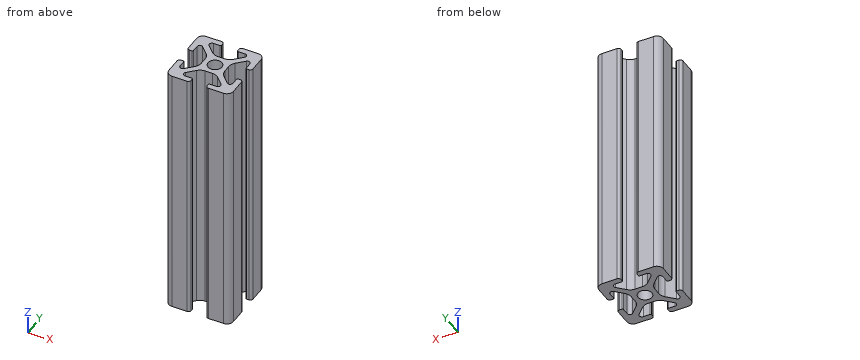
Autodesk Inventor part; units mm, degrees
ref_plane "Startebene" through (0, 0, 0) normal (0, 0, 1) x (1, 0, 0)
ref_plane "Endebene" through (0, 0, 80) normal (0, 0, 1) x (1, 0, 0)
ref_plane "YZ Plane" through (0, 0, 0) normal (1, 0, 0) x (0, 1, 0)
ref_plane "Startebene" through (0, 0, 0) normal (0, 0, 1) x (1, 0, 0)
ref_plane "Endebene" through (0, 0, 80) normal (0, 0, 1) x (1, 0, 0)
sketch "Skizze" plane through (0, 0, 0) normal (0, 0, 1) x (1, 0, 0)
  arc A0 (-4.5287, -3.2559) -> (-3.65, -1.1346) centre (-6.65, -1.1346) ccw
  line L0 (-3.65, -1.1346) -> (-3.65, 1.1346)
  circle A1 centre (0, 0) radius 2.15
  line L1 (1.1346, -3.65) -> (-1.1346, -3.65)
  arc A2 (-1.1346, -3.65) -> (-3.2559, -4.5287) centre (-1.1346, -6.65) ccw
  line L2 (-6.779, -5.5062) -> (-4.5287, -3.2559)
  line L3 (-3.2559, -4.5287) -> (-5.5062, -6.779)
  arc A3 (-2.5, -8.5) -> (-2.8, -8.2) centre (-2.8, -8.5) ccw
  line L4 (-2.5, -8.5) -> (-2.5, -9.2)
  line L5 (-4.9176, -8.2) -> (-2.8, -8.2)
  arc A4 (-5.5062, -6.779) -> (-4.9176, -8.2) centre (-4.9176, -7.3676) ccw
  arc A5 (-3.3, -10) -> (-2.5, -9.2) centre (-3.3, -9.2) ccw
  line L6 (-3.3, -10) -> (-8, -10)
  line L7 (10, -3.3) -> (10, -8)
  line L8 (5.5062, -6.779) -> (3.2559, -4.5287)
  arc A6 (6.779, -5.5062) -> (8.2, -4.9176) centre (7.3676, -4.9176) ccw
  arc A7 (3.2559, -4.5287) -> (1.1346, -3.65) centre (1.1346, -6.65) ccw
  line L9 (4.5287, -3.2559) -> (6.779, -5.5062)
  arc A8 (3.65, -1.1346) -> (4.5287, -3.2559) centre (6.65, -1.1346) ccw
  arc A9 (8.5, -2.5) -> (8.2, -2.8) centre (8.5, -2.8) ccw
  line L10 (3.65, 1.1346) -> (3.65, -1.1346)
  line L11 (8.5, -2.5) -> (9.2, -2.5)
  arc A10 (10, -3.3) -> (9.2, -2.5) centre (9.2, -3.3) ccw
  line L12 (8.2, -4.9176) -> (8.2, -2.8)
  line L13 (2.5, 8.5) -> (2.5, 9.2)
  arc A11 (2.5, 8.5) -> (2.8, 8.2) centre (2.8, 8.5) ccw
  arc A12 (1.1346, 3.65) -> (3.2559, 4.5287) centre (1.1346, 6.65) ccw
  line L14 (-1.1346, 3.65) -> (1.1346, 3.65)
  arc A13 (3.3, 10) -> (2.5, 9.2) centre (3.3, 9.2) ccw
  line L15 (4.9176, 8.2) -> (2.8, 8.2)
  arc A14 (4.5287, 3.2559) -> (3.65, 1.1346) centre (6.65, 1.1346) ccw
  line L16 (3.2559, 4.5287) -> (5.5062, 6.779)
  arc A15 (5.5062, 6.779) -> (4.9176, 8.2) centre (4.9176, 7.3676) ccw
  line L17 (6.779, 5.5062) -> (4.5287, 3.2559)
  line L18 (3.3, 10) -> (8, 10)
  arc A16 (10, 8) -> (8, 10) centre (8, 8) ccw
  line L19 (8.2, 2.8) -> (8.2, 4.9176)
  line L20 (10, 8) -> (10, 3.3)
  arc A17 (8.2, 4.9176) -> (6.779, 5.5062) centre (7.3676, 4.9176) ccw
  line L21 (-2.8, 8.2) -> (-4.9176, 8.2)
  line L22 (-2.5, 9.2) -> (-2.5, 8.5)
  arc A18 (-2.5, 9.2) -> (-3.3, 10) centre (-3.3, 9.2) ccw
  arc A19 (-2.8, 8.2) -> (-2.5, 8.5) centre (-2.8, 8.5) ccw
  arc A20 (-3.65, 1.1346) -> (-4.5287, 3.2559) centre (-6.65, 1.1346) ccw
  arc A21 (-3.2559, 4.5287) -> (-1.1346, 3.65) centre (-1.1346, 6.65) ccw
  arc A22 (4.9176, -8.2) -> (5.5062, -6.779) centre (4.9176, -7.3676) ccw
  arc A23 (8, -10) -> (10, -8) centre (8, -8) ccw
  line L23 (2.8, -8.2) -> (4.9176, -8.2)
  line L24 (8, -10) -> (3.3, -10)
  arc A24 (2.8, -8.2) -> (2.5, -8.5) centre (2.8, -8.5) ccw
  arc A25 (2.5, -9.2) -> (3.3, -10) centre (3.3, -9.2) ccw
  line L25 (2.5, -9.2) -> (2.5, -8.5)
  arc A26 (8.2, 2.8) -> (8.5, 2.5) centre (8.5, 2.8) ccw
  line L26 (9.2, 2.5) -> (8.5, 2.5)
  arc A27 (9.2, 2.5) -> (10, 3.3) centre (9.2, 3.3) ccw
  arc A28 (-4.9176, 8.2) -> (-5.5062, 6.779) centre (-4.9176, 7.3676) ccw
  line L27 (-8, 10) -> (-3.3, 10)
  line L28 (-5.5062, 6.779) -> (-3.2559, 4.5287)
  arc A29 (-8, 10) -> (-10, 8) centre (-8, 8) ccw
  arc A30 (-6.779, 5.5062) -> (-8.2, 4.9176) centre (-7.3676, 4.9176) ccw
  line L29 (-10, 3.3) -> (-10, 8)
  line L30 (-8.2, 4.9176) -> (-8.2, 2.8)
  arc A31 (-8.5, 2.5) -> (-8.2, 2.8) centre (-8.5, 2.8) ccw
  line L31 (-8.5, 2.5) -> (-9.2, 2.5)
  arc A32 (-10, 3.3) -> (-9.2, 2.5) centre (-9.2, 3.3) ccw
  line L32 (-4.5287, 3.2559) -> (-6.779, 5.5062)
  line L33 (-10, -8) -> (-10, -3.3)
  arc A33 (-8.2, -4.9176) -> (-6.779, -5.5062) centre (-7.3676, -4.9176) ccw
  arc A34 (-10, -8) -> (-8, -10) centre (-8, -8) ccw
  line L34 (-10, -8) -> (-10, -3.3)
  arc A35 (-8.2, -2.8) -> (-8.5, -2.5) centre (-8.5, -2.8) ccw
  line L35 (-9.2, -2.5) -> (-8.5, -2.5)
  arc A36 (-9.2, -2.5) -> (-10, -3.3) centre (-9.2, -3.3) ccw
  line L36 (-8.2, -2.8) -> (-8.2, -4.9176)
  dimension "d4" = 4.3
  dimension "d5" = 6.35
  dimension "d6" = 10
  dimension "d7" = 2.5
  dimension "d8" = 5.8
  dimension "d9" = 10.5
  dimension "d10" = 3
  dimension "d11" = 7.5
  dimension "d12" = 12.5
  dimension "d13" = 13.65
  dimension "d14" = 5.7
  dimension "d15" = 10.7
  dimension "d16" = 1.15
  dimension "d17" = 6.15
  dimension "d18" = 1.8
  dimension "d19" = 0.8
  dimension "d20" = 0.3
  dimension "d21" = 2
  dimension "d22" = 0.8324
  dimension "d23" = 45
  dimension "d24" = 90
  dimension "d25" = 90
  dimension "d26" = 1.8
  dimension "d27" = 18.2
  dimension "d28" = 20
  dimension "d29" = 5
  dimension "d30" = 7.5
  dimension "d31" = 1.8
  dimension "d32" = 0.9
  dimension "d33" = 0.9
  dimension "d34" = 20
extrude "Körper" add sketch "Skizze" along normal up to surface (80 mm away) from surface at 0
sketch "Skizze6" plane through (0, 0, 0) normal (0, 0, 1) x (1, 0, 0)
  line L0 (0, 0) -> (10, 0)
ref_plane "Arbeitsebene4" through (0, 0, 0) normal (0, -1, 0) x (1, 0, 0)
sketch "Skizze7" plane through (0, 0, 0) normal (0, -1, 0) x (1, 0, 0)
  line L0 (-2, 0) -> (12, 0)
  line L1 (-2, 80) -> (12, 80)
  dimension "d43" = 80
equation "\"G_OFFSET_START\" = 0"
equation "\"G_OFFSET_END\" = 0"
equation "\"G_L\" = d43"
properties part number "BT001_trajan20_22"
Geometry check sheet. Reference: the model listing, model coordinates, mm. Give positions to 0.01 mm unless a question says otherwise; leave off trailing zeros. Order: outer loops, then holes, each group sorted by start corner. A loop starts at its lowest first (then second) coordinate and runs counter-clockwise, first axis right, second up.
1. Gauge pin test, flat ends, axial feed: pin 1 Ø2.5 at (y, z) = (0, 41.5) entering from +X; pin 2 Ø0.8 at (x, z) = (-9, 50.5) entering from +Y; pin 3 Ø1.1 at (x, z) = (0, 56) entering from -Y; pin 4 Ø4 at (x, y) = (0, 0) entering from +Z. Record the tip position at first contact, or that the pin passes through.
2. Section check A-A, the plane y = 0. Enter the section's corners in (x, z), and give its area (3 significant figures).
3. Thickness scan on L1, parallel to Y at x = 0, z = 40.5; L2, parallel to Y at x = -7.5, z = 6; L3, parallel to Y at x = 3, z = 56. Record the ranges inside material, lowest first.
Values follow:
1. pin 1: stops at x = 3.65
1. pin 2: stops at y = 9.91
1. pin 3: stops at y = -3.65
1. pin 4: passes through
2. outline: (-3.65, 0) - (-2.15, 0) - (-2.15, 80) - (-3.65, 80) - close; (2.15, 0) - (3.65, 0) - (3.65, 80) - (2.15, 80) - close
2. area: 240 mm2
3. L1: y = -3.65 to -2.15, 2.15 to 3.65
3. L2: y = -10 to -5.74, 5.74 to 10
3. L3: y = -9.94 to -8.2, -4.3 to 4.3, 8.2 to 9.94
